Here's how the part is built. I have some questions about the finished solid (model axes, mm). A direction names the side the tool comes from. Round coordinates to 2 decimals unless told otherwise and drop trailing zeros. Loops run counter-clockwise (first coordinate to the right, second up) from the corner with the lowest first, then second, coordinate; pieces in that order, holes last. Notation, with made-up numbers: M -38.75,83 L 12.25,83 A29 ccw 12.25,111 Z; hole C 80.25,-13.5 d7. An arc over 180 degrees is marked long. Answer as CSV lines item,"result".
```python
from build123d import *

# Parameters (mm, degrees)
SKETCH2_W           = 99
SKETCH2_H           = 97
BOSS_EXTRUDE1_DEPTH = 3
BOSS_EXTRUDE2_DEPTH = 27
SKETCH5_R           = 1.75
CUT_EXTRUDE1_DEPTH  = 4
FILLET1_R           = 2


with BuildPart() as part:
    # Sketch2 → Boss-Extrude1 (new body)
    with BuildSketch(Plane(origin=(0, 0, 0), x_dir=(1, 0, 0), z_dir=(0, 1, 0))):
        with Locations((49.5, 48.5)):
            Rectangle(SKETCH2_W, SKETCH2_H)
    extrude(amount=BOSS_EXTRUDE1_DEPTH)

    # Sketch4 → Boss-Extrude2 (add)
    with BuildSketch(Plane(origin=(0, 3, 0), x_dir=(1, 0, 0), z_dir=(0, 1, 0))):
        Polygon((17.5, 97), (89, 97), (89, 0), (17.5, 0), (0, 0), (0, 1.5), (17.5, 1.5), align=None)
    extrude(amount=BOSS_EXTRUDE2_DEPTH)

    # Sketch5 → Cut-Extrude1 (cut, through all)
    with BuildSketch(Plane(origin=(0, 3, 0), x_dir=(1, 0, 0), z_dir=(0, 1, 0))):
        with Locations((3.5, 91.5)):
            Circle(SKETCH5_R)
        with BuildLine():
            Line((96, 8.25), (99, 8.25))
            Line((99, 8.25), (99, 4.75))
            Line((99, 4.75), (96, 4.75))
            ThreePointArc((96, 4.75), (94.25, 6.5), (96, 8.25))
        make_face()
    extrude(amount=-CUT_EXTRUDE1_DEPTH, mode=Mode.SUBTRACT)

    # Fillet1
    fillet1_edges = [part.edges().sort_by_distance(p)[0] for p in [
        (0, 1.5, -97),
        (99, 1.5, -97),
    ]]
    fillet(fillet1_edges, radius=FILLET1_R)


solid = part.part
```
1. I want a section at A-A, the plane x = 3.5. Please give me the cut outline in (y, z).
Evaluation:
outline,"M 0,-97 L 3,-97 L 3,-93.25 L 0,-93.25 Z; M 0,-89.75 L 3,-89.75 L 3,-1.5 L 30,-1.5 L 30,0 L 0,0 Z"
2. I want a section at C-C, the plane z = -73. Please give me the cut outline in (x, y).
Evaluation:
outline,"M 0,0 L 99,0 L 99,3 L 89,3 L 89,30 L 17.5,30 L 17.5,3 L 0,3 Z"
3. I want a section at B-B, the plane z = -91.5. Please give me the cut outline in (x, y), and give its area (3 significant figures).
Evaluation:
outline,"M 0,0 L 1.75,0 L 1.75,3 L 0,3 Z; M 5.25,0 L 99,0 L 99,3 L 89,3 L 89,30 L 17.5,30 L 17.5,3 L 5.25,3 Z"
area,"2,220 mm²"
4. Which directions (+Z, -Z, +X, -X, +Y, -Y) give clear straight access to the entire face, cutting with the end or side of a thin tool? Please do faces 1 (the flat face through (0, 2, -47)), 2 (the flat face through (9, 16, -1.5)), 3 (the flat face through (89, 16, -49)), 4 (the flat face through (97, 2, -8.25)), 5 (the flat face through (49, 15, 0)).
Evaluation:
face 1,"+Z, -Z, -X, +Y, -Y"
face 2,"-Z, -X, +Y"
face 3,"+Z, -Z, +X, +Y"
face 4,"+X, +Y, -Y"
face 5,"+Z, +X, -X, +Y, -Y"
5. For P1, Ø4.5, axis at x = 3.5, z = -91.5, coming from the +Y side; P2, Ø13.5, axis at y = 17, z = -57.5, coming from the +X side; P3, Ø2, axis at y = 13.5, z = -28.5, coming from the -X side, each with a flat end and sliding along its axis, tell me the tip position at first contact or that it passes through.
Evaluation:
P1,"stops at y = 3"
P2,"stops at x = 89"
P3,"stops at x = 17.5"
6. I want a section at D-D, the plane y = 11. Please give me the cut outline in (x, z), and give its area (3 significant figures).
Evaluation:
outline,"M 0,-1.5 L 17.5,-1.5 L 17.5,-97 L 89,-97 L 89,0 L 0,0 Z"
area,"6,960 mm²"
7. If I drill on line 1 (Z direction, x = 3.5, y = 1.2); line 2 (X direction, y = 2.15, z = -91.5); line 3 (X direction, y = 23.5, z = -14), over which ranges is the centre line in solid material (lowest first)? Write a range as [from, to].
Evaluation:
line 1,"z = [-97, -93.25], [-89.75, 0]"
line 2,"x = [0, 1.75], [5.25, 99]"
line 3,"x = [17.5, 89]"
